```python
from build123d import *

# Parameters (mm, degrees)
SKETCH1_W           = 250
SKETCH1_H           = 13.5
SKETCH1_R           = 2.5
BOSS_EXTRUDE1_DEPTH = 2
SKETCH3_W           = 250
SKETCH3_H           = 1
BOSS_EXTRUDE2_DEPTH = 5.5
FILLET1_R           = 1
FILLET2_R           = 0.5


with BuildPart() as part:
    # Sketch1 → Boss-Extrude1 (new body)
    with BuildSketch(Plane(origin=(0, 0, 0), x_dir=(1, 0, 0), z_dir=(0, 1, 0))):
        Rectangle(SKETCH1_W, SKETCH1_H)
        with Locations(Location((0, 0, 0), (0, 0, 270))):
            Circle(SKETCH1_R, mode=Mode.SUBTRACT)
        with Locations(Location((-50, 0, 0), (0, 0, 270))):
            Circle(SKETCH1_R, mode=Mode.SUBTRACT)
        with Locations(Location((-100, 0, 0), (0, 0, 270))):
            Circle(SKETCH1_R, mode=Mode.SUBTRACT)
        with Locations(Location((50, 0, 0), (0, 0, 270))):
            Circle(SKETCH1_R, mode=Mode.SUBTRACT)
        with Locations(Location((100, 0, 0), (0, 0, 270))):
            Circle(SKETCH1_R, mode=Mode.SUBTRACT)
        with Locations(Location((115, 0, 0), (0, 0, 270))):
            Circle(SKETCH1_R, mode=Mode.SUBTRACT)
    extrude(amount=BOSS_EXTRUDE1_DEPTH)

    # Sketch3 → Boss-Extrude2 (add)
    with BuildSketch(Plane(origin=(0, 2, 0), x_dir=(1, 0, 0), z_dir=(0, 1, 0))):
        with Locations((0, 6.25)):
            Rectangle(SKETCH3_W, SKETCH3_H)
        with Locations((0, -6.25)):
            Rectangle(SKETCH3_W, SKETCH3_H)
    extrude(amount=BOSS_EXTRUDE2_DEPTH)

    # Fillet1
    fillet1_edges = [part.edges().sort_by_distance(p)[0] for p in [
        (0, 2, -5.75),
        (0, 0, 6.75),
        (0, 2, 5.75),
        (-125, 0, 0),
        (0, 0, -6.75),
        (125, 0, 0),
    ]]
    fillet(fillet1_edges, radius=FILLET1_R)

    # Fillet2
    fillet2_edges = [part.edges().sort_by_distance(p)[0] for p in [
        (-125, 7.5, -6.25),
        (0, 7.5, -5.75),
        (125, 7.5, -6.25),
        (0, 7.5, -6.75),
        (-125, 7.5, 6.25),
        (0, 7.5, 6.75),
        (125, 7.5, 6.25),
        (0, 7.5, 5.75),
    ]]
    fillet(fillet2_edges, radius=FILLET2_R - 0.0001)  # a hair under: the kernel refuses the full size


solid = part.part
```
Geometry check sheet. Reference: the model listing, model coordinates, mm. A direction names the side the tool comes from. Coordinates: 2 decimals unless noted, no trailing zeros. Order: outer loops, then holes, each group sorted by start corner. A loop starts at its lowest first (then second) coordinate and runs counter-clockwise, first axis right, second up. Notation, with made-up numbers: (15.5, 10.5) - (30.5, 10.5) arc R13 cw to (30.5, 23.5) - close; hole circle Ø7 at (76, 68). An arc over 180 degrees is marked (long way). Use one line per item in the form item = value.
1. Section check B-B (z = 0). State how many separate pieces and enclosed holes the cut face has, then the cut area to 3 significant figures.
Here are the results:
separate_pieces = 7
enclosed_holes = 0
area = 440 mm²
2. Gauge pin test, flat ends, axial feed: pin 1 (2 mm diameter, centred on x = 15, z = 2, fed in from +Y); pin 2 (3 mm diameter, centred on x = -100, z = 0, fed in from +Y). Record the tip position at first contact, or that the pin passes through.
Here are the results:
pin_1 = 2
pin_2 = through
3. Section check A-A (y = 4.75). Record the boundary of the cut face in (x, z).
Here are the results:
outline = (-125, -6.75) - (125, -6.75) - (125, -5.75) - (-125, -5.75) - close; (-125, 5.75) - (125, 5.75) - (125, 6.75) - (-125, 6.75) - close
4. Access from +Z, -Z, +X, -X, +Y, -Y to the whole of each face (thin tool, end or side, straight path). Record for faces 1 (the face through (117.48, 0.99, -0.33)), 2 (the face through (-2, 2, -2)).
Here are the results:
face_1 = +Y, -Y
face_2 = +X, -X, +Y
5. Scan lines: line 1 (Z direction, x = 88, y = 6.25); line 2 (Y direction, x = 111.5, z = -2); line 3 (Z direction, x = 72.5, y = 2.75). Record each from-to range of solid material in increasing order.
Here are the results:
line_1 = -6.75 to -5.75, 5.75 to 6.75
line_2 = 0 to 2
line_3 = -6.75 to -5.72, 5.72 to 6.75
6. Draft check along Z on faces 3 (the face through (-2, 0, 2)), 4 (the face through (-97.52, 0.99, -0.33)), 5 (the face through (-2, 4, 6.75)). Enter one of: pulls with the +Z half, pulls with the -Z half, needs draft (parallel to the pull), parting line crosses it, or undercut.
Here are the results:
face_3 = needs draft
face_4 = undercut
face_5 = pulls with the +Z half
